Autodesk Inventor part; units mm, degrees
ref_plane "YZ Plane" through (0, 0, 0) normal (1, 0, 0) x (0, 1, 0)
ref_plane "XZ Plane" through (0, 0, 0) normal (0, 1, 0) x (-1, 0, 0)
ref_plane "XY Plane" through (0, 0, 0) normal (0, 0, 1) x (1, 0, 0)
sketch "Sketch1" plane through (0, 0, 0) normal (0, 1, 0) x (-1, 0, 0)
  line L0 (0, 0) -> (252, 0)
  line L1 (252, 0) -> (252, -155)
  line L2 (252, -155) -> (0, -155)
  line L3 (0, -155) -> (0, 0)
  dimension "d0" = 252
  dimension "d1" = 155
extrude "Plate1" add sketch "Sketch1" along normal blind 1
sketch "Sketch2" plane through (-1, 1, 0) normal (1, 0, 0) x (0, 1, 0)
  line L0 (0, -155) -> (0, 0)
  line L1 (0, 0) -> (-61, 0)
  line L2 (-61, 0) -> (-61, -155)
  line L3 (-61, -155) -> (0, -155)
edge flange "Flange1" height 61 angle 90 thickness 1 bend radius 1 thickness toward (1, 0, 0) relief tear relief width 1 relief depth 0.5 edges at (0, 0, -77.5) wall of the first edge with corners at (-1, 1, -155) (-1, 1, 0) (-1, -60, 0) (-1, -60, -155)
bend "Bend1"
corner "Corner1"
sketch "Sketch3" plane through (-251, 1, -155) normal (-1, 0, 0) x (0, -1, 0)
  line L0 (0, 155) -> (0, 0)
  line L1 (0, 0) -> (61, 0)
  line L2 (61, 0) -> (61, 155)
  line L3 (61, 155) -> (0, 155)
edge flange "Flange2" height 61 angle 90 thickness 1 bend radius 1 thickness toward (-1, 0, 0) relief tear relief width 1 relief depth 0.5 edges at (-252, 0, -77.5) wall of the first edge with corners at (-251, 1, 0) (-251, 1, -155) (-251, -60, -155) (-251, -60, 0)
bend "Bend2"
corner "Corner2"
sketch "Sketch4" plane through (0, 1, 0) normal (0, 1, 0) x (1, 0, 0)
  line L0 (0, 155) -> (0, 0)
  line L1 (0, 0) -> (0, 77.5)
  line L2 (0, 77.5) -> (-71, 77.5)
  circle A0 centre (-71, 77.5) radius 47
  line L3 (-71, 77.5) -> (-71, 133) construction
  line L4 (-71, 77.5) -> (-71, 22) construction
  circle A1 centre (-71, 133) radius 2.25
  circle A2 centre (-71, 22) radius 2.25
  dimension "d23" = 77.5
  dimension "d24" = 71
  dimension "d25" = 94
  dimension "d26" = 55.5
  dimension "d27" = 55.5
  dimension "d28" = 4.5
  dimension "d29" = 4.5
extrude "Extrusion1" cut sketch "Sketch4" against normal through all
sketch "Sketch5" plane through (0, 1, 0) normal (0, 1, 0) x (1, 0, 0)
  line L0 (-252, 0) -> (-252, 155)
  line L1 (0, 155) -> (0, 0)
  line L2 (-250, 155) -> (-2, 155)
  line L3 (-2, 0) -> (-250, 0)
  point P0 (-177, 147)
  point P1 (-75, 147)
  point P2 (-177, 8)
  point P3 (-75, 8)
  dimension "d32" = 75
  dimension "d33" = 75
  dimension "d34" = 8
  dimension "d35" = 8
hole "Hole1" at (-177, 1, -147) at (-75, 1, -147) at (-177, 1, -8) at (-75, 1, -8) direction (0, -1, 0) diameter 4.5 end through all
sketch "Sketch6" plane through (0, -60, 0) normal (1, 0, 0) x (0, 0, -1)
  line L0 (0, 0) -> (0, 59)
  line L1 (155, 0) -> (0, 0)
  line L2 (155, 59) -> (155, 0)
  point P0 (0, 60)
  point P1 (8, 24)
  point P2 (77.5, 7)
  point P3 (147, 24)
  dimension "d43" = 77.5
  dimension "d44" = 7
  dimension "d45" = 8
  dimension "d46" = 8
  dimension "d47" = 24
  dimension "d48" = 24
hole "Hole2" at (0, -36, -8) at (0, -53, -77.5) at (0, -36, -147) direction (-1, 0, 0) diameter 4.5 end through all
sketch "Sketch7" plane through (0, -60, 0) normal (1, 0, 0) x (0, 0, -1)
  line L0 (155, 60) -> (0, 60)
  line L1 (0, 59) -> (155, 59)
  line L2 (77.5, 59) -> (42.5, 59)
  line L3 (42.5, 59) -> (42.5, 14)
  line L4 (42.5, 14) -> (112.5, 14)
  line L5 (112.5, 14) -> (112.5, 59)
  point P0 (49.5, 52)
  point P1 (49.5, 21)
  point P2 (105.5, 21)
  point P3 (105.5, 52)
  dimension "d57" = 35
  dimension "d58" = 45
  dimension "d59" = 70
  dimension "d60" = 7
  dimension "d61" = 7
  dimension "d62" = 7
  dimension "d63" = 7
hole "Hole3" at (0, -8, -49.5) at (0, -39, -49.5) at (0, -39, -105.5) at (0, -8, -105.5) direction (-1, 0, 0) diameter 6 depth 1
equation "\"d41\" = Thickness"
equation "\"d54\" = Thickness"
equation "\"d69\" = Thickness"
equation "\"d2\" = Thickness"
equation "\"d3\" = BendReliefWidth"
equation "\"d4\" = BendReliefDepth"
equation "\"d5\" = MinimumRemnant"
equation "\"d6\" = TransitionRadius"
equation "\"d9\" = BendRadius"
equation "\"d10\" = CornerReliefSize"
equation "\"d11\" = GapSize"
equation "\"d12\" = JacobiRadiusSize"
equation "\"d13\" = BendReliefWidth"
equation "\"d14\" = BendReliefDepth"
equation "\"d15\" = MinimumRemnant"
equation "\"d16\" = TransitionRadius"
equation "\"d19\" = BendRadius"
equation "\"d20\" = CornerReliefSize"
equation "\"d21\" = GapSize"
equation "\"d22\" = JacobiRadiusSize"
equation "\"BendRadius\" = Thickness"
equation "\"BendReliefWidth\" = Thickness"
equation "\"BendReliefDepth\" = 0.5 * Thickness"
equation "\"CornerReliefSize\" = 4 * Thickness"
equation "\"MinimumRemnant\" = 2 * Thickness"
equation "\"TransitionRadius\" = BendRadius"
equation "\"JacobiRadiusSize\" = BendRadius"
equation "\"GapSize\" = Thickness"
properties part number "tapa_v7" material "Steel, Carbon"
Check sheet for the modelled part. Datum: model origin and axes. Units: mm. A direction names the side the tool comes from. Round coordinates to 2 decimals unless told otherwise and drop trailing zeros. Loops run counter-clockwise (first coordinate to the right, second up) from the corner with the lowest first, then second, coordinate; pieces in that order, holes last. Notation, with made-up numbers: M 69,13 L 106,13 A21 cw 106,36 Z; hole C -31,87.5 d7. An arc over 180 degrees is marked long. One line per question, with ' | ' between items. Start each with the question number.
Item 1: Set-up check for faces 1 (the face through (-1, -30, -76)), 2 (the face through (-0.5, -6.2, -103.1)), 3 (the face through (-252, -31, -79)): record each of +Z, -Z, +X, -X, +Y, -Y from which the full face is reachable in a straight line by a thin tool's end or side.
Item 2: Section check C-C (y = -45). Record the boundary of the cut face in (x, z).
Item 3: Release check for a two-part mould opening along Z. For faces 4 (the face through (-0.51, -41.03, -103.29)), 5 (the face through (-251, -30, -79)), 6 (the face through (-27.584, 0.507, -59.499)) record: released by +Z, released by -Z, zero draft, split by the parting line, or undercut.
Item 4: Section check A-A (y = -8). Record the boundary of the cut face in (x, z), and give its area (3 significant figures).
Item 5: Scan lines: probe 1 along Z at (x, y) = (-177, 0.3); probe 2 along X at (y, z) = (-23, -96); probe 3 along X at (y, z) = (0.3, -8). Record each from-to range of solid material in increasing order.
Item 6: Section check B-B (x = -57.5). Record the boundary of the cut face in (y, z).
Item 7: Section check D-D (z = -86). Record the boundary of the cut face in (x, y) (3 decimals), and give its area (3 significant figures).
Item 8: Gauge pin test, flat end, axial feed: pin 1 Ø5 at (y, z) = (-39, -49.5) entering from +X. Record the tip position at first contact, or that the pin passes through.
Worked out:
1) face 1: +Z, -Z, -Y | face 2: +X | face 3: +Z, -Z, -X, +Y, -Y
2) outline: M -252,-155 L -251,-155 L -251,0 L -252,0 Z; M -1,-155 L 0,-155 L 0,0 L -1,0 Z
3) face 4: undercut | face 5: zero draft | face 6: undercut
4) outline: M -252,-155 L -251,-155 L -251,0 L -252,0 Z; M -1,-155 L 0,-155 L 0,-108.5 L -1,-108.5 Z; M -1,-102.5 L 0,-102.5 L 0,-52.5 L -1,-52.5 Z; M -1,-46.5 L 0,-46.5 L 0,0 L -1,0 Z | area: 298 mm^2
5) probe 1: -155 to -149.25, -144.75 to -10.25, -5.75 to 0 | probe 2: -252 to -251, -1 to 0 | probe 3: -251.52 to -179.25, -174.75 to -77.25, -72.75 to -0.48
6) outline: M 0,-155 L 1,-155 L 1,-122.52 L 0,-122.52 Z; M 0,-32.48 L 1,-32.48 L 1,0 L 0,0 Z
7) outline: M -252,-60 L -251,-60 L -251,-1 A1 cw -250,0 L -117.225,0 L -117.225,1 L -250,1 A2 ccw -252,-1 Z; M -24.775,0 L -2,0 A1 cw -1,-1 L -1,-60 L 0,-60 L 0,-1 A2 ccw -2,1 L -24.775,1 Z | area: 278 mm^2
8) pin 1: x = -251
